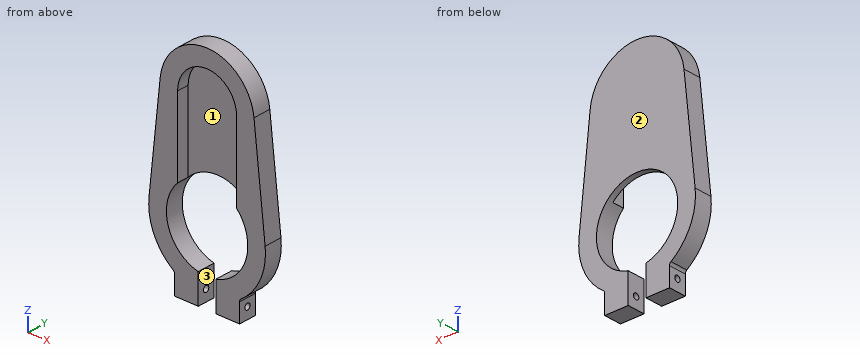
from build123d import *

# Parameters (mm, degrees)
F1_DEPTH = 19.05
F3_DEPTH = 12.7
F5_D     = 6.35
F6_R     = 3.81


with BuildPart() as f1:
    # F0 (on Front) → F1 (new body)
    with BuildSketch(Plane.XZ):
        with BuildLine():
            ThreePointArc((-9.525, -42.767144), (0, 43.815), (9.525, -42.767144))
            Line((9.525, -42.767144), (9.525, -74.517144))
            Line((9.525, -74.517144), (34.925, -74.517144))
            Line((34.925, -74.517144), (34.925, -52.270954))
            ThreePointArc((34.925, -52.270954), (56.930482, -26.663241), (62.513799, 6.63575))
            Line((62.513799, 6.63575), (50.516201, 119.662222))
            ThreePointArc((50.516201, 119.662222), (0, 165.1), (-50.516201, 119.662222))
            Line((-50.516201, 119.662222), (-62.513799, 6.63575))
            ThreePointArc((-62.513799, 6.63575), (-56.930482, -26.663241), (-34.925, -52.270954))
            Line((-34.925, -52.270954), (-34.925, -74.517144))
            Line((-34.925, -74.517144), (-9.525, -74.517144))
            Line((-9.525, -74.517144), (-9.525, -42.767144))
        make_face()
    extrude(amount=F1_DEPTH)

    # F2 (on face) → F3 (cut)
    with BuildSketch(Plane.XZ.offset(19.05)):
        with BuildLine():
            Line((31.75, 12.7), (31.75, 114.3))
            ThreePointArc((31.75, 114.3), (0, 146.05), (-31.75, 114.3))
            Line((-31.75, 114.3), (-31.75, 12.7))
            Line((-31.75, 12.7), (31.75, 12.7))
        make_face()
    extrude(amount=-F3_DEPTH, mode=Mode.SUBTRACT)

    # F5 (through all)
    with Locations(Plane.YZ.offset(34.925)):
        with Locations((-9.525, -62.430954)):
            Hole(F5_D / 2)

    # F6
    f6_edges = [f1.edges().sort_by_distance(p)[0] for p in [
        (34.925, -9.525, -52.270954),
        (-34.925, -9.525, -52.270954),
    ]]
    fillet(f6_edges, radius=F6_R)


solid = f1.part
For this review, take the finished solid that the model builds, in its own axes (mm). Face numbers are marked on the shaded views. A direction names the side the tool comes from. Round coordinates to 2 decimals unless told otherwise and drop trailing zeros. Loops run counter-clockwise (first coordinate to the right, second up) from the corner with the lowest first, then second, coordinate; pieces in that order, holes last. Notation, with made-up numbers: (44, 9.5) - (59, 9.5) arc R23 ccw to (59, 24.5) - close; hole circle Ø10 at (16, -18.75). An arc over 180 degrees is marked (long way). Use one line per item in the form item = value.
Item 1: Consider section C-C on y = -4. Write out the cut boundary in (x, z) (3 decimals), then the cut area to 3 significant figures.
Answers:
outline = (-62.514, 6.636) arc R62.865 ccw to (-36.522, -51.168) arc R3.81 cw to (-34.925, -54.269) - (-34.925, -74.517) - (-9.525, -74.517) - (-9.525, -42.767) arc R43.815 cw (long way) to (9.525, -42.767) - (9.525, -74.517) - (34.925, -74.517) - (34.925, -54.269) arc R3.81 cw to (36.522, -51.168) arc R62.865 ccw to (62.514, 6.636) - (50.516, 119.662) arc R50.8 ccw to (-50.516, 119.662) - close
area = 17,800 mm^2
Item 2: Consider section D-D on x = 0. Write out the cut boundary in (y, z) (3 decimals), then the cut area to 3 significant figures.
Answers:
outline = (-19.05, 146.05) - (-6.35, 146.05) - (-6.35, 43.815) - (0, 43.815) - (0, 165.1) - (-19.05, 165.1) - close
area = 1,010 mm^2
Item 3: For line 1 (X direction, y = -7, z = -57.5) (3 decimals); line 2 (Y direction, x = -0.5, z = 135); line 3 (Z direction, x = -37, y = -4), list the stretches that pass through material, from the lowest coordinate up.
Answers:
line_1 = -34.925 to -9.525, 9.525 to 34.925
line_2 = -6.35 to 0
line_3 = -50.82 to -23.47, 23.47 to 149.11
Item 4: Clearance check with flat-ended pins moving along their axes: P1, Ø4, axis at y = -9.52, z = -62.43, coming from the -X side; P2, Ø8.5, axis at y = -9.52, z = -62.43, coming from the +X side (3 decimals); P3, Ø6, axis at y = -2, z = 89, coming from the +X side; P4, Ø9.5, axis at y = -11, z = -65, coming from the -X side (3 decimals). State where each tip first meets the part, or that it passes through.
Answers:
P1 = through
P2 = 34.925
P3 = 54.09
P4 = -34.925
Item 5: Tool access review of the marked faces 1, 2 and 3: name each direction out of +Z, -Z, +X, -X, +Y, -Y from which nothing blocks a thin tool from reaching the whole face with its end or side.
Answers:
face_1 = -Y
face_2 = +Z, -Z, +X, -X, +Y
face_3 = -Z, +Y, -Y
Item 6: Consider section A-A on z = 0. Write out the cut boundary in (x, y) (3 decimals).
Answers:
outline = (-62.865, -19.05) - (-43.815, -19.05) - (-43.815, 0) - (-62.865, 0) - close; (43.815, -19.05) - (62.865, -19.05) - (62.865, 0) - (43.815, 0) - close
Item 7: Consider section B-B on x = 17. Write out the cut boundary in (y, z) (3 decimals).
Answers:
outline = (-19.05, -74.517) - (0, -74.517) - (0, -40.383) - (-19.05, -40.383) - close; (-19.05, 141.115) - (-6.35, 141.115) - (-6.35, 40.383) - (0, 40.383) - (0, 162.171) - (-19.05, 162.171) - close; hole circle Ø6.35 at (-9.525, -62.431)
